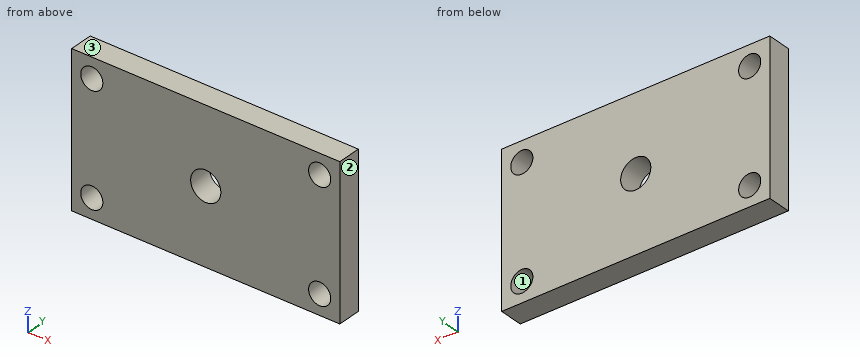
from build123d import *

# Parameters (mm, degrees)
F0_W     = 80
F0_H     = 45
F1_DEPTH = 7
F3_D     = 6.6
F5_D     = 9


with BuildPart() as f1:
    # F0 (on Front) → F1 (new body)
    with BuildSketch(Plane.XZ):
        Rectangle(F0_W, F0_H)
    extrude(amount=F1_DEPTH)

    # F3 (through all)
    with Locations(Plane.XZ.offset(7)):
        with Locations((-34, 16.5), (-34, -16.5), (34, -16.5), (34, 16.5)):
            Hole(F3_D / 2)

    # F5 (through all)
    with Locations(Plane.XZ.offset(7)):
        with Locations((0, 0)):
            Hole(F5_D / 2)


solid = f1.part
The model under review builds one solid part; all positions refer to its coordinate system, in mm. Face numbers are marked on the shaded views. Give positions to 0.01 mm unless a question says otherwise; leave off trailing zeros. Order: outer loops, then holes, each group sorted by start corner. A loop starts at its lowest first (then second) coordinate and runs counter-clockwise, first axis right, second up. Notation, with made-up numbers: M -24.75,3 L 7.25,3 A12 cw 7.25,21 Z; hole C -1.75,43.25 d10. An arc over 180 degrees is marked long. One line per question, with ' | ' between items. Start each with the question number.
1) Wall thickness on L1, parallel to Z at x = 34, y = -3.5; L2, parallel to Z at x = 0, y = -3; L3, parallel to X at y = -5.5, z = 15.5: over which ranges is each line inside the solid? List them lowest first. Write a range as from..to.
2) Mouldability with a two-part tool opening along Z and no side actions: class the marked faces 1, 2 and 3 as pulls with the +Z half, pulls with the -Z half, needs draft (parallel to the pull), parting line crosses it, or undercut.
3) Consider section D-D, the plane y = -5.25. Give the boundary of the cut face in (x, z).
4) Consider section C-C, the plane x = 0. Give the boundary of the cut face in (y, z), then the cut area to 3 significant figures.
5) Consider section B-B, the plane z = 0. Give the boundary of the cut face in (x, y), then the cut area to 3 significant figures.
6) Consider section A-A, the plane z = 16.5. Give the boundary of the cut face in (x, y).
Found:
1) L1: z = -22.5..-19.8, -13.2..13.2, 19.8..22.5 | L2: z = -22.5..-4.5, 4.5..22.5 | L3: x = -40..-37.14, -30.86..30.86, 37.14..40
2) face 1: undercut | face 2: needs draft | face 3: pulls with the +Z half
3) outline: M -40,-22.5 L 40,-22.5 L 40,22.5 L -40,22.5 Z; hole C -34,-16.5 d6.6; hole C -34,16.5 d6.6; hole C 0,0 d9; hole C 34,-16.5 d6.6; hole C 34,16.5 d6.6
4) outline: M -7,-22.5 L 0,-22.5 L 0,-4.5 L -7,-4.5 Z; M -7,4.5 L 0,4.5 L 0,22.5 L -7,22.5 Z | area: 252 mm²
5) outline: M -40,-7 L -4.5,-7 L -4.5,0 L -40,0 Z; M 4.5,-7 L 40,-7 L 40,0 L 4.5,0 Z | area: 497 mm²
6) outline: M -40,-7 L -37.3,-7 L -37.3,0 L -40,0 Z; M -30.7,-7 L 30.7,-7 L 30.7,0 L -30.7,0 Z; M 37.3,-7 L 40,-7 L 40,0 L 37.3,0 Z
